Here's how the part is built. I have some questions about the finished solid (model axes, mm). Round coordinates to 2 decimals unless told otherwise and drop trailing zeros. Loops run counter-clockwise (first coordinate to the right, second up) from the corner with the lowest first, then second, coordinate; pieces in that order, holes last. Notation, with made-up numbers: M 87.5,8.25 L 133.5,8.25 A22 ccw 133.5,44.25 Z; hole C 89.5,70 d6. An arc over 180 degrees is marked long. Answer as CSV lines item,"result".
```python
from build123d import *

# Parameters (mm, degrees)
BOSS_EXTRUDE1_DEPTH = 1.524
SKETCH2_W           = 1.524
SKETCH2_H           = 5.96660367
CUT_EXTRUDE3_DEPTH  = 135.253240476


with BuildPart() as part:
    # Sketch1 → Boss-Extrude1 (new body)
    with BuildSketch(Plane.XY):
        with BuildLine():
            Line((52.749938031, 70.131845749), (64.371465794, 71.381472391))
            Line((64.371465794, 71.381472391), (64.371465794, 72.905472391))
            Line((64.371465794, 72.905472391), (58.560701913, 72.905472391))
            ThreePointArc((58.560701913, 72.905472391), (68.751288874, 77.18302052), (79.665108288, 78.924866217))
            ThreePointArc((79.665108288, 78.924866217), (87.51605356, 79.864840631), (94.759202069, 76.693453987))
            ThreePointArc((94.759202069, 76.693453987), (96.985502082, 75.005001445), (97.746636466, 72.316515219))
            ThreePointArc((97.746636466, 72.316515219), (100.280996817, 69.637712422), (101.428823049, 66.133220769))
            ThreePointArc((101.428823049, 66.133220769), (102.504441665, 63.756169776), (104.763633539, 62.451034186))
            ThreePointArc((104.763633539, 62.451034186), (105.815523966, 61.94348794), (105.834353574, 60.775702811))
            ThreePointArc((105.834353574, 60.775702811), (107.593647808, 59.110829557), (107.413611762, 56.69535731))
            ThreePointArc((107.413611762, 56.69535731), (104.915486102, 51.493806045), (99.669748601, 49.089849838))
            ThreePointArc((99.669748601, 49.089849838), (97.93078373, 50.558543058), (97.277362732, 52.738932839))
            ThreePointArc((97.277362732, 52.738932839), (96.275148178, 55.045205965), (94.377694548, 56.69535731))
            ThreePointArc((94.377694548, 56.69535731), (94.341947265, 57.697226126), (93.911436782, 58.602587774))
            ThreePointArc((93.911436782, 58.602587774), (93.31755476, 58.718236433), (92.715544448, 58.657787675))
            ThreePointArc((92.715544448, 58.657787675), (92.668251349, 57.985085863), (92.857476868, 57.337816162))
            ThreePointArc((92.857476868, 57.337816162), (92.437007408, 57.816991843), (92.308352921, 58.441373075))
            ThreePointArc((92.308352921, 58.441373075), (91.998939648, 58.544100362), (91.680077423, 58.476156637))
            ThreePointArc((91.680077423, 58.476156637), (91.653768646, 58.005927685), (91.779444676, 57.552041185))
            ThreePointArc((91.779444676, 57.552041185), (91.306585055, 57.779976677), (91.03290283, 58.22791512))
            ThreePointArc((91.03290283, 58.22791512), (90.50619799, 58.023829811), (90.170237064, 57.569738347))
            ThreePointArc((90.170237064, 57.569738347), (89.940738286, 57.243637966), (89.778811712, 56.879233065))
            ThreePointArc((89.778811712, 56.879233065), (89.744476135, 57.449042317), (89.940738286, 57.985085863))
            ThreePointArc((89.940738286, 57.985085863), (89.626896453, 58.063679483), (89.308840631, 58.00439924))
            ThreePointArc((89.308840631, 58.00439924), (87.283822401, 55.344960061), (84.23724791, 53.969569406))
            ThreePointArc((84.23724791, 53.969569406), (82.119422653, 54.881253432), (80.968584276, 56.879233065))
            ThreePointArc((80.968584276, 56.879233065), (80.728221934, 58.038765282), (80.225263479, 59.110829557))
            ThreePointArc((80.225263479, 59.110829557), (79.990436789, 59.199276584), (79.74821764, 59.133730156))
            ThreePointArc((79.74821764, 59.133730156), (78.063200875, 56.684963047), (75.700496179, 54.881253432))
            ThreePointArc((75.700496179, 54.881253432), (74.814943925, 54.724384759), (73.92939167, 54.881253432))
            ThreePointArc((73.92939167, 54.881253432), (72.689360724, 57.184690211), (71.555199225, 59.542056419))
            ThreePointArc((71.555199225, 59.542056419), (70.53318823, 60.33987445), (69.280379472, 60.673776077))
            ThreePointArc((69.280379472, 60.673776077), (66.074534091, 56.320096732), (62.023949735, 52.738932839))
            ThreePointArc((62.023949735, 52.738932839), (62.018158819, 52.275784748), (62.122280661, 51.824455233))
            ThreePointArc((62.122280661, 51.824455233), (61.681410811, 52.454602529), (61.618245883, 53.221063245))
            ThreePointArc((61.618245883, 53.221063245), (59.29856558, 51.252524719), (56.623131886, 49.804037512))
            ThreePointArc((56.623131886, 49.804037512), (56.143365032, 49.668212915), (55.855452098, 50.075313269))
            ThreePointArc((55.855452098, 50.075313269), (55.634539123, 50.152406549), (55.491712516, 49.967078524))
            ThreePointArc((55.491712516, 49.967078524), (54.711546462, 49.408479108), (53.79819099, 49.114414214))
            ThreePointArc((53.79819099, 49.114414214), (53.781075658, 48.622130566), (53.534831875, 48.19551584))
            ThreePointArc((53.534831875, 48.19551584), (53.542028616, 48.644457223), (53.48523445, 49.089849838))
            ThreePointArc((53.48523445, 49.089849838), (53.3082991, 49.130815552), (53.13136375, 49.089849838))
            ThreePointArc((53.13136375, 49.089849838), (53.00604404, 48.779905646), (52.700390386, 48.644457223))
            ThreePointArc((52.700390386, 48.644457223), (52.714349204, 48.082434529), (52.379221144, 47.631043855))
            ThreePointArc((52.379221144, 47.631043855), (52.460297524, 48.107812169), (52.379221144, 48.584580484))
            ThreePointArc((52.379221144, 48.584580484), (52.12852371, 48.695194866), (51.864428363, 48.622130566))
            ThreePointArc((51.864428363, 48.622130566), (51.051818187, 47.620090335), (49.775293704, 47.433261089))
            ThreePointArc((49.775293704, 47.433261089), (49.651036263, 47.688587532), (49.62023506, 47.970868935))
            ThreePointArc((49.62023506, 47.970868935), (48.780471907, 47.225294105), (47.727759637, 46.834294287))
            ThreePointArc((47.727759637, 46.834294287), (47.331273993, 46.008852436), (46.594544028, 45.464992092))
            ThreePointArc((46.594544028, 45.464992092), (46.877970347, 46.066432963), (46.906161005, 46.730712185))
            ThreePointArc((46.906161005, 46.730712185), (43.798654282, 45.811386919), (40.571228797, 45.519014346))
            ThreePointArc((40.571228797, 45.519014346), (37.159419224, 45.129203066), (33.725626021, 45.090971596))
            ThreePointArc((33.725626021, 45.090971596), (33.068999074, 44.320201948), (32.178585471, 43.838114389))
            ThreePointArc((32.178585471, 43.838114389), (32.418564973, 44.441560177), (32.417226894, 45.090971596))
            ThreePointArc((32.417226894, 45.090971596), (31.873442168, 44.988363543), (31.332044302, 45.102899962))
            ThreePointArc((31.332044302, 45.102899962), (30.887683341, 44.585264996), (30.259078376, 44.320201948))
            ThreePointArc((30.259078376, 44.320201948), (30.326970235, 44.626264328), (30.531184649, 44.864129748))
            ThreePointArc((30.531184649, 44.864129748), (29.980102952, 45.010427729), (29.429021254, 44.864129748))
            ThreePointArc((29.429021254, 44.864129748), (29.340661001, 44.432357132), (28.989623083, 44.165884794))
            ThreePointArc((28.989623083, 44.165884794), (28.864149038, 44.515007271), (28.989623083, 44.864129748))
            ThreePointArc((28.989623083, 44.864129748), (28.628355518, 44.84783713), (28.30893512, 44.678277961))
            ThreePointArc((28.30893512, 44.678277961), (27.079850519, 43.991023465), (25.955408412, 43.143322074))
            ThreePointArc((25.955408412, 43.143322074), (26.282852866, 43.874201462), (26.857193183, 44.432357132))
            ThreePointArc((26.857193183, 44.432357132), (25.328745526, 44.244978672), (23.791384091, 44.333198545))
            ThreePointArc((23.791384091, 44.333198545), (25.414182464, 44.809450383), (27.079850519, 45.102435547))
            ThreePointArc((27.079850519, 45.102435547), (23.023366565, 45.343696153), (19.045869652, 46.176034458))
            ThreePointArc((19.045869652, 46.176034458), (16.652090777, 47.015108036), (14.752643777, 48.696275152))
            ThreePointArc((14.752643777, 48.696275152), (14.640422349, 48.961729487), (14.752643777, 49.227183822))
            ThreePointArc((14.752643777, 49.227183822), (15.539561177, 50.138860369), (16.635728101, 50.637670147))
            ThreePointArc((16.635728101, 50.637670147), (35.605852794, 58.693330375), (52.749938031, 70.131845749))
        make_face()
    extrude(amount=BOSS_EXTRUDE1_DEPTH)

    # Sketch2 → Cut-Extrude3 (cut, through all)
    with BuildSketch(Plane.XY.offset(1.524)):
        with Locations((72.435845658, 59.192908392)):
            Rectangle(SKETCH2_W, SKETCH2_H)
        Polygon((106.940547802, 54.636029996), (106.397081003, 53.169068481), (104.827290354, 54.203248276), (105.665710767, 55.475894028), align=None)
    extrude(amount=-CUT_EXTRUDE3_DEPTH, mode=Mode.SUBTRACT)


with BuildPart() as cut_extrude3_kept_piece:
    # of the separate pieces the step leaves, the one the design keeps (cut_extrude3_pieces_kept)
    add(part.part.solids().sort_by_distance((16.635728101, 50.637670147, 0))[0])


solid = cut_extrude3_kept_piece.part
```
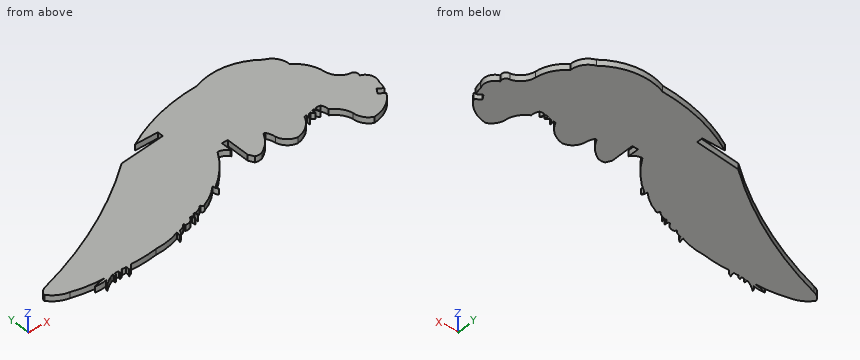
1. I want a section at B-B, the plane y = 74. Please give me the cut outline in (x, z).
Evaluation:
outline,"M 60.6,0 L 97.5,0 L 97.5,1.52 L 60.6,1.52 Z"
2. I want a section at A-A, the plane x = 43.5. Please give me the cut outline in (y, z), and give its area (3 significant figures).
Evaluation:
outline,"M 45.76,0 L 63.39,0 L 63.39,1.52 L 45.76,1.52 Z"
area,"26.9 mm²"
3. For P1, Ø6, axis at x = 73.5, y = 70.5, coming from the -Z side; P2, Ø0.8, axis at y = 60, z = 0.5, coming from the -X side; P3, Ø0.8, axis at x = 73, z = 0.5, coming from the -Y side, each with a flat end and sliding along its axis, tell me the tip position at first contact or that it passes through.
Evaluation:
P1,"stops at z = 0"
P2,"stops at x = 37.25"
P3,"stops at y = 55.83"
4. If I drill on line 1 (X direction, y = 60, z = 0.8); line 2 (Y direction, x = 63.5, z = 1.45); line 3 (Y direction, x = 61, z = 1.2), over which ranges is the centre line in solid material (lowest first)? Write a range as [from, to].
Evaluation:
line 1,"x = [37.96, 68.87], [71.07, 71.67], [73.2, 107.04]"
line 2,"y = [53.87, 71.29], [72.91, 75.34]"
line 3,"y = [52.61, 71.02], [72.91, 74.2]"
